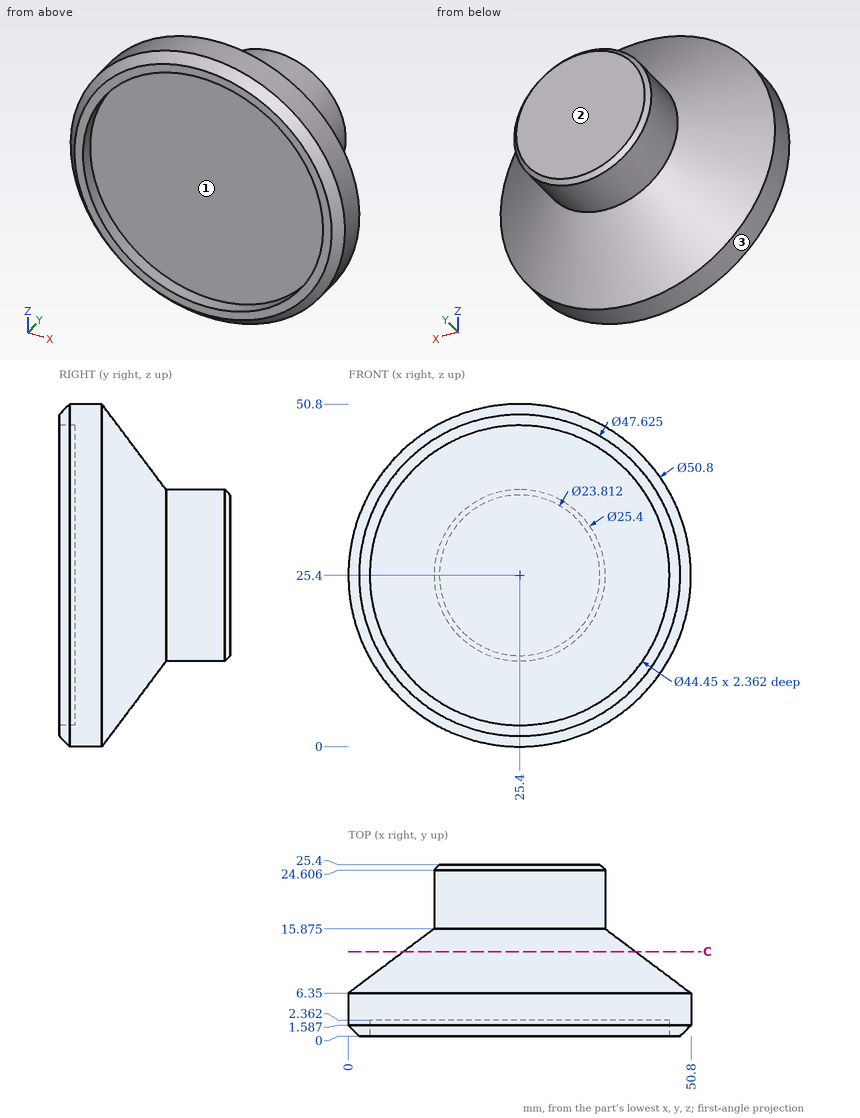
For this review, use the dimensioned drawing (mm, ordinates from the lowest corner) and the shaded views. Round coordinates to 2 decimals unless told otherwise and drop trailing zeros. Write each loop counter-clockwise with the first axis right and the second up, starting at its lowest first coordinate (ties: lowest second). Pieces come first, ordered by that corner, then holes. Notation, with made-up numbers: (63.5, 32) - (89.5, 32) arc R25 cw to (89.5, 62) - close; hole circle Ø1 at (8, 71.25). An arc over 180 degrees is marked (long way). Answer as CSV lines item,"result". Start each with the question number.
(1) For pin 1 Ø10 at (y, z) = (8.5, 33) entering from +X; pin 2 Ø1.5 at (x, z) = (31, 35) entering from -Y; pin 3 Ø1 at (y, z) = (2.5, 22.5) entering from +X, all flat-tipped, find the tip position at first contact; note any pin that passes through.
(2) To check wall thickness, follow line 1 (Z direction, x = 24, y = 2); line 2 (Y direction, x = 32, z = 26); line 3 (X direction, y = 2, z = 6) (1 decimal). State the ranges of each line that lie inside material, in increasing order.
(3) We need section C-C on y = 12.5. State the section outline as (x, z) points.
(4) Draft analysis for pull direction X (two halves, no side actions). For the marked faces 1, 2 and 3, state which applies: pulls with the +X half, pulls with the -X half, needs draft (parallel to the pull), parting line crosses it, or undercut.
Worked answers:
1,pin 1,"x = 50.61"
1,pin 2,"y = 2.36"
1,pin 3,"x = 50.69"
2,line 1,"0.04 to 3.22, 47.58 to 50.76"
2,line 2,"2.36 to 25.4"
2,line 3,"9 to 14.6, 36.2 to 41.8"
3,outline,"circle Ø34.4 at (25.4, 25.4)"
4,face 1,"undercut"
4,face 2,"needs draft"
4,face 3,"parting line crosses it"
